```python
from build123d import *

# Parameters (mm, degrees)
SKETCH_1_W      = 37
SKETCH_1_H      = 30
EXTRUDE_1_DEPTH = 34
SKETCH_2_R      = 12
EXTRUDE_2_DEPTH = 8
SKETCH_3_R      = 11.25
EXTRUDE_3_DEPTH = 10


with BuildPart() as part:
    # Эскиз1 → Бобышка-Вытянуть1 (new body)
    with BuildSketch(Plane(origin=(0, 0, 0), x_dir=(1, 0, 0), z_dir=(0, 1, 0))):
        Rectangle(SKETCH_1_W, SKETCH_1_H)
    extrude(amount=-EXTRUDE_1_DEPTH)

    # Эскиз2 → Бобышка-Вытянуть2 (add)
    with BuildSketch(Plane(origin=(0, 0, 0), x_dir=(1, 0, 0), z_dir=(0, 1, 0))):
        Circle(SKETCH_2_R)
    extrude(amount=EXTRUDE_2_DEPTH)

    # Эскиз3 → Бобышка-Вытянуть3 (add)
    with BuildSketch(Plane(origin=(0, 8, 0), x_dir=(1, 0, 0), z_dir=(0, 1, 0))):
        Circle(SKETCH_3_R)
    extrude(amount=EXTRUDE_3_DEPTH)

    # Эскиз4 → Повернуть1 (revolve)
    with BuildSketch(Plane(origin=(0, 0, 0), x_dir=(0, 0, -1), z_dir=(1, 0, 0))):
        with BuildLine():
            Line((0, 18), (0, 39))
            ThreePointArc((0, 39), (10.307764064, 37.731056256), (20, 34))
            Line((20, 34), (20, 31))
            Line((20, 31), (11.5, 31))
            Line((11.5, 31), (11.5, 26))
            Line((11.5, 26), (7.5, 26))
            Line((7.5, 26), (7.5, 18))
            Line((7.5, 18), (0, 18))
        make_face()
    revolve(axis=Axis((0, -965.379937914, 0), (0, 1, 0)))


solid = part.part
```
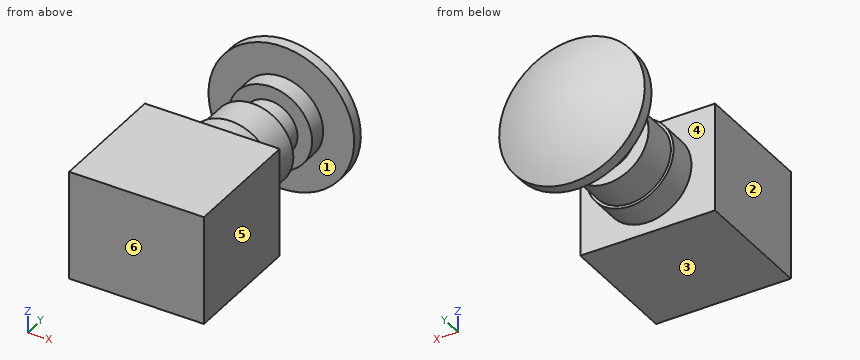
Verification items for the finished model (mm, model axes). Face numbers are marked on the shaded views. A direction names the side the tool comes from. Give positions to 0.01 mm unless a question says otherwise; leave off trailing zeros. Write each loop counter-clockwise with the first axis right and the second up, starting at its lowest first coordinate (ties: lowest second). Pieces come first, ordered by that corner, then holes. Notation, with made-up numbers: M 72.5,1 L 124.5,1 A17 ccw 124.5,7 Z; hole C 71,1 d6. An arc over 180 degrees is marked long. One line per question, with ' | ' between items.
1) Section check D-D on x = 0. Enter the section's corners in (y, z).
Result:
outline: M -34,-15 L 0,-15 L 0,-12 L 8,-12 L 8,-11.25 L 18,-11.25 L 18,-7.5 L 26,-7.5 L 26,-11.5 L 31,-11.5 L 31,-20 L 34,-20 A42.5 ccw 34,20 L 31,20 L 31,11.5 L 26,11.5 L 26,7.5 L 18,7.5 L 18,11.25 L 8,11.25 L 8,12 L 0,12 L 0,15 L -34,15 Z
2) Section check B-B on z = 0. Enter the section's corners in (x, y), plus the area to 3 significant figures.
Result:
outline: M -20,31 L -11.5,31 L -11.5,26 L -7.5,26 L -7.5,18 L -11.25,18 L -11.25,8 L -12,8 L -12,0 L -18.5,0 L -18.5,-34 L 18.5,-34 L 18.5,0 L 12,0 L 12,8 L 11.25,8 L 11.25,18 L 7.5,18 L 7.5,26 L 11.5,26 L 11.5,31 L 20,31 L 20,34 A42.5 ccw -20,34 Z | area: 2,160 mm2
3) Mould release check, pull along Y, two halves, no side actions. Record for the marked faces 4, 5 and 6: released by +Y, released by -Y, zero draft, split by the parting line, or undercut.
Result:
face 4: undercut | face 5: zero draft | face 6: released by -Y
4) Section check A-A on x = 16. Enter the section's corners in (y, z).
Result:
outline: M -34,-15 L 0,-15 L 0,15 L -34,15 Z; M 31,-12 L 34,-12 A39.37 ccw 34,12 L 31,12 Z
5) Set-up check for the marked faces 1, 2 and 3: record each of +Z, -Z, +X, -X, +Y, -Y from which the full face is reachable in a straight line by a thin tool's end or side.
Result:
face 1: none | face 2: +Z, -Z, -X, -Y | face 3: -Z, +X, -X, -Y
6) Section check C-C on z = -9. Enter the section's corners in (x, y), plus the area to 3 significant figures.
Result:
outline: M -18.5,-34 L 18.5,-34 L 18.5,0 L 7.94,0 L 7.94,8 L 6.75,8 L 6.75,18 L -6.75,18 L -6.75,8 L -7.94,8 L -7.94,0 L -18.5,0 Z; M -17.86,31 L -7.16,31 L -7.16,26 L 7.16,26 L 7.16,31 L 17.86,31 L 17.86,34 A41.54 ccw -17.86,34 Z | area: 1,800 mm2
7) Thickness scan on line 1 along X through (y, z) = (-29.5, -4); line 2 along Z through (x, y) = (-10, -14.5); line 3 along Y through (x, z) = (-2.5, 8.5). Record the ranges inside material, lowest first. Write a range as [from, to].
Result:
line 1: x = [-18.5, 18.5] | line 2: z = [-15, 15] | line 3: y = [-34, 18], [26, 38.07]
8) Gauge pin test, flat ends, axial feed: pin 1 Ø10 at (x, y) = (8, 2) entering from +Z; pin 2 Ø1.5 at (x, z) = (13, 11) entering from +Y; pin 3 Ø12 at (x, y) = (-13.5, -1.5) entering from -Z; pin 4 Ø19 at (x, z) = (5, 0.5) entering from +Y. Record the tip position at first contact, or that the pin passes through.
Result:
pin 1: stops at z = 15 | pin 2: stops at y = 35.76 | pin 3: stops at z = -15 | pin 4: stops at y = 39
